For this review, use the dimensioned drawing (mm, ordinates from the lowest corner) and the shaded views. Coordinates: 2 decimals unless noted, no trailing zeros. Write each loop counter-clockwise with the first axis right and the second up, starting at its lowest first coordinate (ties: lowest second). Pieces come first, ordered by that corner, then holes. Notation, with made-up numbers: (-11, 59) - (-2, 59) arc R7 ccw to (-2, 64) - close; hole circle Ø8 at (79.5, -31.75). An arc over 180 degrees is marked (long way). Answer as a JSON object with one key per item and string values.
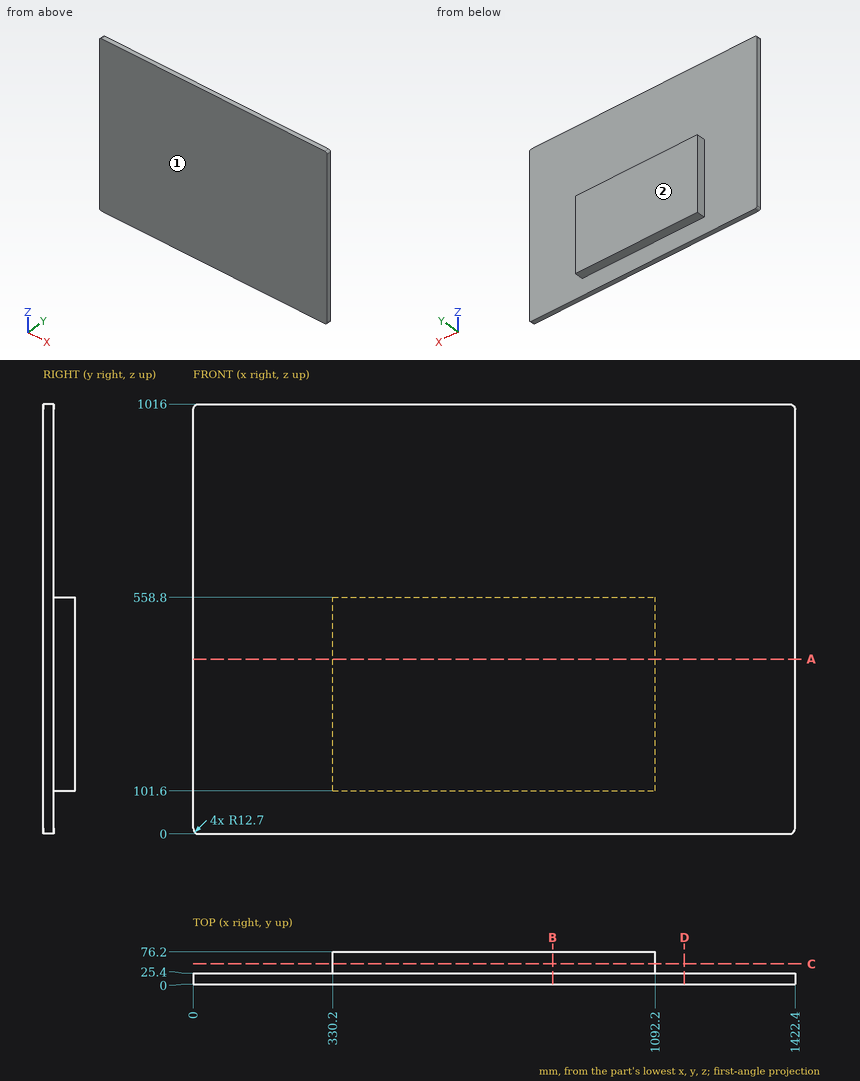
(1) The part is to be moulded in two halves that separate along Y. For the marked faces 1 and 2, say which applies: pulls with the +Y half, pulls with the -Y half, needs draft (parallel to the pull), parting line crosses it, or undercut.
Solved:
{"face 1": "pulls with the -Y half", "face 2": "pulls with the +Y half"}
(2) Take a section at D-D, the plane x = 1161. Write out the cut boundary in (y, z).
Solved:
{"outline": "(0, 0) - (25.4, 0) - (25.4, 1016) - (0, 1016) - close"}
(3) Take a section at B-B, the plane x = 849.5. Write out the cut boundary in (y, z).
Solved:
{"outline": "(0, 0) - (25.4, 0) - (25.4, 101.6) - (76.2, 101.6) - (76.2, 558.8) - (25.4, 558.8) - (25.4, 1016) - (0, 1016) - close"}
(4) To check wall thickness, follow line 1 (Z direction, x = 570, y = 42); line 2 (Y direction, x = 394.5, z = 74.5); line 3 (X direction, y = 60, z = 527). State the ranges of each line that lie inside material, in increasing order. Write a range as from..to.
Solved:
{"line 1": "z = 101.6..558.8", "line 2": "y = 0..25.4", "line 3": "x = 330.2..1092.2"}
(5) For pin 1 (8 mm diameter, centred on x = 535.5, y = 51, fed in from -Z); pin 2 (4 mm diameter, centred on x = 203, z = 269.5, fed in from +Y); pin 3 (15 mm diameter, centred on y = 38.5, z = 443.5, fed in from +X), all flat-tipped, find the tip position at first contact; note any pin that passes through.
Solved:
{"pin 1": "stops at z = 101.6", "pin 2": "stops at y = 25.4", "pin 3": "stops at x = 1092.2"}
(6) Take a section at C-C, the plane y = 48. Write out the cut boundary in (x, z).
Solved:
{"outline": "(330.2, 101.6) - (1092.2, 101.6) - (1092.2, 558.8) - (330.2, 558.8) - close"}
(7) Take a section at A-A, the plane z = 413. Write out the cut boundary in (x, y).
Solved:
{"outline": "(0, 0) - (1422.4, 0) - (1422.4, 25.4) - (1092.2, 25.4) - (1092.2, 76.2) - (330.2, 76.2) - (330.2, 25.4) - (0, 25.4) - close"}
